Autodesk Inventor part; units mm, degrees
ref_plane "YZ Plane" through (0, 0, 0) normal (1, 0, 0) x (0, 1, 0)
ref_plane "XZ Plane" through (0, 0, 0) normal (0, 1, 0) x (-1, 0, 0)
ref_plane "XY Plane" through (0, 0, 0) normal (0, 0, 1) x (1, 0, 0)
sketch "Sketch1" plane through (0, 0, 0) normal (0, 1, 0) x (-1, 0, 0)
  circle A0 centre (0, 0) radius 20
  dimension "d0" = 40
extrude "Extrusion1" add sketch "Sketch1" along normal blind 10
sketch "Sketch2" plane through (0, 10, 0) normal (0, 1, 0) x (1, 0, 0)
  circle A0 centre (0, 0) radius 20
  circle A1 centre (0, 0) radius 6
  dimension "d3" = 12
extrude "Extrusion2" cut sketch "Sketch2" against normal blind 10 contours A1
sketch "Sketch3" plane through (0, 10, 0) normal (0, 1, 0) x (1, 0, 0)
  circle A0 centre (-12.593, 0) radius 1.5
  circle A1 centre (12.593, 0) radius 1.5
  dimension "d7" = 3
  dimension "d8" = 3
extrude "Extrusion3" cut sketch "Sketch3" against normal blind 10
sketch "Sketch6" plane through (0, 10, 0) normal (0, 1, 0) x (1, 0, 0)
  circle A0 centre (0, 0) radius 6
  circle A1 centre (0, 0) radius 20
  circle A2 centre (0, 0) radius 5
  dimension "d11" = 10
extrude "Extrusion4" add sketch "Sketch6" against normal blind 10 contours A0
sketch "Sketch7" plane through (0, 10, 0) normal (0, 1, 0) x (1, 0, 0)
  circle A0 centre (0, 0) radius 5
  circle A1 centre (0, 0) radius 20
  circle A2 centre (0, 0) radius 3
  dimension "d14" = 6
extrude "Extrusion5" add sketch "Sketch7" against normal blind 2 contours A0
sketch "Sketch8" plane through (0, 10, 0) normal (0, 1, 0) x (1, 0, 0)
  circle A0 centre (0, 0) radius 20
  line L0 (9, 17.8606) -> (9, 7.8606)
  line L1 (9, 7.8606) -> (-9, 7.8606)
  line L2 (-9, 7.8606) -> (-9, 17.8606)
  line L3 (-9, 17.8606) -> (9, 7.8606) construction
  line L4 (9, 17.8606) -> (-9, 7.8606) construction
  arc A1 (9, 17.8606) -> (-9, 17.8606) centre (0, 0) ccw
  point P0 (0, 12.8606)
  dimension "d17" = 18
  dimension "d18" = 10
extrude "Extrusion6" cut sketch "Sketch8" against normal blind 10 contours L0 L1 L2 A0 picked at (0, 11.9071)
sketch "Sketch9" plane through (0, 10, 0) normal (0, 1, 0) x (1, 0, 0)
  line L0 (-9, 7.8606) -> (9, 7.8606)
  line L1 (9, 7.8606) -> (9, 5.8606)
  line L2 (9, 5.8606) -> (-9, 5.8606)
  line L3 (-9, 5.8606) -> (-9, 7.8606)
  dimension "d21" = 18
  dimension "d25" = 2
extrude "Extrusion7" cut sketch "Sketch9" against normal blind 10
sketch "Sketch10" plane through (0, 0, 0) normal (0, -1, 0) x (1, 0, 0)
  circle A0 centre (0, 0) radius 5
extrude "Extrusion8" add sketch "Sketch10" against normal blind 8
sketch "Sketch11" plane through (0, 8, 0) normal (0, 1, 0) x (1, 0, 0)
  circle A0 centre (0, 0) radius 3
extrude "Extrusion9" cut sketch "Sketch11" against normal blind 8
sketch "Sketch12" plane through (0, 10, 0) normal (0, 1, 0) x (1, 0, 0)
  circle A0 centre (0, 0) radius 3
  arc A1 (-9, 17.8606) -> (9, 17.8606) centre (0, 0) ccw
  circle A2 centre (0, 0) radius 2
  dimension "d32" = 4
extrude "Extrusion10" add sketch "Sketch12" against normal blind 10
fillet "Fillet1" radius 1 2 edges at (9, 5, -5.8606) (-9, 5, -5.8606)
fillet "Fillet2" radius 4 2 edges at (0, 0, 20) (0, 10, 20)
properties part number "ruka_lozisko"
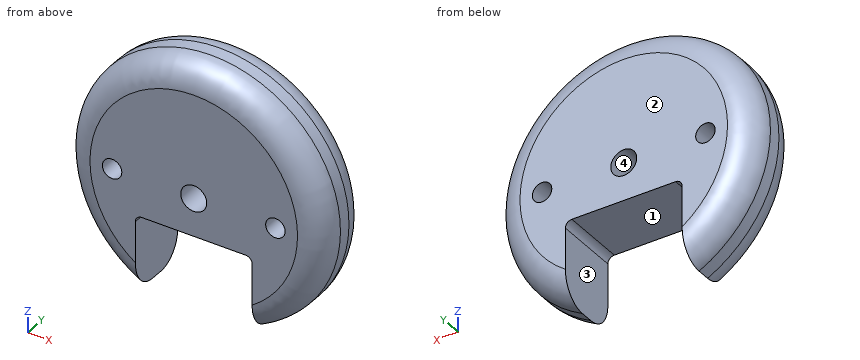
Could you check a few things on this model? Use its own coordinates, in mm. Face numbers are marked on the shaded views. A direction names the side the tool comes from. Give positions to 0.01 mm unless a question says otherwise; leave off trailing zeros. Order: outer loops, then holes, each group sorted by start corner. A loop starts at its lowest first (then second) coordinate and runs counter-clockwise, first axis right, second up.
1. For the marked faces 3 and 4, which set-ups out of +Z, -Z, +X, -X, +Y, -Y let a thin tool reach every point of the face, with its end or its side?
2. Suppose I cut it at A-A (z = 0). List the corners of the cut face in (x, y) for me.
3. We'd pull the mould along X, two halves only. Please class the marked faces 1 and 2: pulls with the +X half, pulls with the -X half, needs draft (parallel to the pull), parting line crosses it, or undercut.
4. I need wall thicknesses on L1, parallel to X at y = 4, z = 0; L2, parallel to X at y = 6.75, z = 0; L3, parallel to Z at x = -0.5, y = 0.5. Which ranges of each line are inside material? Lowest first, please.
5. Suppose I cut it at C-C (y = 2.5). List the corners of the cut face in (x, z) for me.
6. Will these pins go through, and if not, where does the flat tip stop? P1, Ø3, axis at y = 7, z = -14.5, coming from the +X side; P2, Ø10, axis at x = -3.5, z = -11, coming from the +Y side; P3, Ø1.5, axis at x = -13.5, y = 7.5, coming from the -Z side; P4, Ø5, axis at x = 4, y = 6, coming from the -Z side.
7. Suppose I cut it at B-B (x = 0). List the corners of the cut face in (y, z) for me, plus the area to 3 significant figures.
Solved:
1. face 3: -Z, +Y, -Y
1. face 4: +Y, -Y
2. outline: (-20, 4) arc R4 ccw to (-16, 0) - (-14.09, 0) - (-14.09, 10) - (-16, 10) arc R4 ccw to (-20, 6) - close; (-11.09, 0) - (-2, 0) - (-2, 10) - (-11.09, 10) - close; (2, 0) - (11.09, 0) - (11.09, 10) - (2, 10) - close; (14.09, 0) - (16, 0) arc R4 ccw to (20, 4) - (20, 6) arc R4 ccw to (16, 10) - (14.09, 10) - close
3. face 1: undercut
3. face 2: needs draft
4. L1: x = -20 to -14.09, -11.09 to -2, 2 to 11.09, 14.09 to 20
4. L2: x = -19.93 to -14.09, -11.09 to -2, 2 to 11.09, 14.09 to 19.93
4. L3: z = -5.86 to -1.94, 1.94 to 17.93
5. outline: (-9, -17.53) - (-9, -6.86) arc R1 cw to (-8, -5.86) - (8, -5.86) arc R1 cw to (9, -6.86) - (9, -17.53) arc R19.71 ccw (long way) to start; hole circle Ø3 at (-12.59, 0); hole circle Ø4 at (0, 0); hole circle Ø3 at (12.59, 0)
6. P1: stops at x = 15.09
6. P2: passes through
6. P3: stops at z = -15.12
6. P4: stops at z = -5.86
7. outline: (0, -5.86) - (10, -5.86) - (10, -2) - (0, -2) - close; (0, 2) - (10, 2) - (10, 16) arc R4 ccw to (6, 20) - (4, 20) arc R4 ccw to (0, 16) - close
7. area: 212 mm2
